For this review, take the finished solid that the model builds, in its own axes (mm). Face numbers are marked on the shaded views. A direction names the side the tool comes from. Coordinates: 2 decimals unless noted, no trailing zeros. Order: outer loops, then holes, each group sorted by start corner. A loop starts at its lowest first (then second) coordinate and runs counter-clockwise, first axis right, second up. Notation, with made-up numbers: M 53.5,55.25 L 67.5,55.25 A9 ccw 67.5,69.25 Z; hole C 78,51 d1. An arc over 180 degrees is marked long. Use CSV: the item, a comma, the result in double quotes.
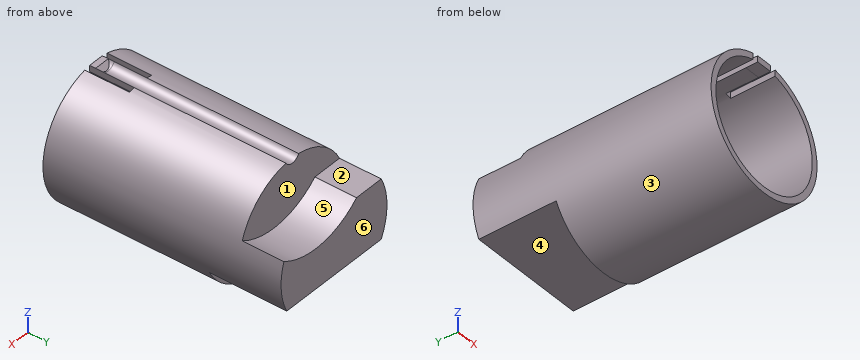
```python
from build123d import *

# Parameters (mm, degrees)
SKETCH1_R           = 11
BOSS_EXTRUDE1_DEPTH = 40
CUT_EXTRUDE1_START  = -13
CUT_EXTRUDE1_DEPTH  = 13
CUT_EXTRUDE2_START  = -7
CUT_EXTRUDE2_DEPTH  = 7
CUT_EXTRUDE3_DEPTH  = 37.482872694
SKETCH6_R           = 10
CUT_EXTRUDE4_DEPTH  = 25
SKETCH7_W           = 1
SKETCH7_H           = 7.5
CUT_EXTRUDE5_DEPTH  = 7
SKETCH8_W           = 2.630926858
SKETCH8_H           = 1.007959983
BOSS_EXTRUDE2_DEPTH = 2
CHAMFER1_SIZE       = 1


with BuildPart() as part:
    # Sketch1 → Boss-Extrude1 (new body)
    with BuildSketch(Plane(origin=(0, 0, 0), x_dir=(1, 0, 0), z_dir=(0, 1, 0))):
        with Locations(Location((0, 0, 0), (0, 0, 270))):
            Circle(SKETCH1_R)
    extrude(amount=BOSS_EXTRUDE1_DEPTH)

    # Sketch2 → Cut-Extrude1 (cut)
    with BuildSketch(Plane(origin=(0, 40, 0), x_dir=(1, 0, 0), z_dir=(0, 1, 0)).offset(CUT_EXTRUDE1_START)):
        with BuildLine():
            Line((-9.797958971, 5), (9.797958971, 5))
            ThreePointArc((9.797958971, 5), (0, 11), (-9.797958971, 5))
        make_face()
    extrude(amount=CUT_EXTRUDE1_DEPTH, mode=Mode.SUBTRACT)

    # Sketch3 → Cut-Extrude2 (cut)
    with BuildSketch(Plane(origin=(0, 40, 0), x_dir=(1, 0, 0), z_dir=(0, 1, 0)).offset(CUT_EXTRUDE2_START)):
        with BuildLine():
            Line((-9.797958971, -5), (-4.683015841, -5))
            ThreePointArc((-4.683015841, -5), (2.619314521, -1.734147983), (10.406466307, -3.564471772))
            ThreePointArc((10.406466307, -3.564471772), (0.779586825, -10.972339968), (-9.797958971, -5))
        make_face()
    extrude(amount=CUT_EXTRUDE2_DEPTH, mode=Mode.SUBTRACT)

    # Sketch4 → Cut-Extrude3 (cut, through all)
    with BuildSketch(Plane(origin=(0, 33, 0), x_dir=(1, 0, 0), z_dir=(0, 1, 0))):
        with BuildLine():
            ThreePointArc((1.315463429, -10.921060203), (0, -10.120855836), (-1.315463429, -10.921060203))
            ThreePointArc((-1.315463429, -10.921060203), (0, -11), (1.315463429, -10.921060203))
        make_face()
    extrude(amount=-CUT_EXTRUDE3_DEPTH, mode=Mode.SUBTRACT)

    # Sketch6 → Cut-Extrude4 (cut)
    with BuildSketch(Plane.XZ):
        with Locations(Location((0, 0, 0), (0, 0, 270))):
            Circle(SKETCH6_R)
    extrude(amount=-CUT_EXTRUDE4_DEPTH, mode=Mode.SUBTRACT)

    # Sketch7 → Cut-Extrude5 (cut)
    with BuildSketch(Plane.XY.offset(12)):
        with Locations((-1.815463429, 3.75)):
            Rectangle(SKETCH7_W, SKETCH7_H)
        with Locations((1.815463429, 3.75)):
            Rectangle(SKETCH7_W, SKETCH7_H)
    extrude(amount=-CUT_EXTRUDE5_DEPTH, mode=Mode.SUBTRACT)

    # Sketch8 → Boss-Extrude2 (add)
    with BuildSketch(Plane.XZ):
        with Locations((0, 10.417080212)):
            Rectangle(SKETCH8_W, SKETCH8_H)
    extrude(amount=-BOSS_EXTRUDE2_DEPTH)

    # Chamfer1
    # the kernel refuses this chamfer: 1 mm, written as the material it takes off along each edge
    with BuildSketch(Plane(origin=(-3.887146417, 2, 10.921060203), x_dir=(-9.448986822191204e-15, 0.02749587661058651, -0.9996219169112968), z_dir=(1, 0, 0))) as chamfer1_piece_1_section:
        Polygon((CHAMFER1_SIZE * 0.999621916911, -CHAMFER1_SIZE * 0.0274958766106), (-CHAMFER1_SIZE * 0.0274958766106, -CHAMFER1_SIZE * 0.999621916911), (0, 0), align=None)
    chamfer1_piece_1 = extrude(amount=7.774292833, mode=Mode.PRIVATE)
    chamfer1_piece_1 = chamfer1_piece_1 & Plane(origin=(0, 1.631347526, 11.602209324), x_dir=(0.8880145347419771, 0, -0.45981538261240235), z_dir=(0, 1, 0)) * Cylinder(1.481353488, 20, mode=Mode.PRIVATE)
    add(chamfer1_piece_1, mode=Mode.SUBTRACT)


solid = part.part
```
Item 1: For the marked faces 1, 2, 3 and 4, list the 3-axis set-ups (+Z, -Z, +X, -X, +Y, -Y) from which the entire face can be reached by the end or side of a thin tool; tool diameter is ignored.
Solutions:
face 1,"+Z, +Y"
face 2,"+Z, +X, -X, +Y"
face 3,"+Y, -Y"
face 4,"-Z, +X, -X, +Y"
Item 2: Clearance check with flat-ended pins moving along their axes: pin 1 Ø0.8 at (x, z) = (1.5, 10.5) entering from -Y; pin 2 Ø1 at (x, z) = (-6, 8) entering from +Y; pin 3 Ø2.5 at (x, y) = (-7, 36) entering from +Z; pin 4 Ø1.5 at (x, z) = (-1, 2) entering from -Y. State where each tip first meets the part, or that it passes through.
Solutions:
pin 1,"y = 0"
pin 2,"y = 33"
pin 3,"z = 5"
pin 4,"y = 25"
Item 3: Draft analysis for pull direction Y (two halves, no side actions). For the marked faces 5 and 6, state which applies: released by +Y, released by -Y, zero draft, split by the parting line, or undercut.
Solutions:
face 5,"zero draft"
face 6,"released by +Y"
Item 4: Add section B-B on z = 0. State the section outline as (x, y) points, and give its area (3 significant figures).
Solutions:
outline,"M -11,0 L -10,0 L -10,25 L 10,25 L 10,0 L 11,0 L 11,40 L -11,40 Z"
area,"380 mm^2"
Item 5: Add section C-C on x = -9. State the section outline as (y, z) points, and give its area (3 significant figures).
Solutions:
outline,"M 0,-6.32 L 27,-6.32 L 27,-5 L 40,-5 L 40,5 L 33,5 L 33,6.32 L 0,6.32 L 0,4.36 L 25,4.36 L 25,-4.36 L 0,-4.36 Z"
area,"262 mm^2"
Item 6: Add section D-D on y = 17. State the section outline as (x, z) points.
Solutions:
outline,"M -1.32,10.92 A11 ccw long 1.32,10.92 A1.48 cw Z; hole C 0,0 d20"
Item 7: To check wall thickness, follow line 1 along X through (y, z) = (7.75, 0); line 2 along Y through (x, z) = (2.5, -7.25); line 3 along Y through (x, z) = (4.75, 1.25). State the ranges of each line that lie inside material, in increasing order. Write a range as [from, to].
Solutions:
line 1,"[-11, -10], [10, 11]"
line 2,"[25, 27]"
line 3,"[25, 40]"
Item 8: Add section A-A on y = 7. State the section outline as (x, z) points.
Solutions:
outline,"M -2.32,9.73 L -2.32,10.75 A11 ccw long 2.32,10.75 L 2.32,9.73 A10 cw long Z; M -1.32,9.91 A10 cw 1.32,9.91 L 1.32,10.92 A1.48 cw -1.32,10.92 Z"
